Could you check a few things on this model? Use its own coordinates, in mm. A direction names the side the tool comes from. Give positions to 0.01 mm unless a question says otherwise; leave off trailing zeros. Order: outer loops, then holes, each group sorted by start corner. A loop starts at its lowest first (then second) coordinate and runs counter-clockwise, first axis right, second up. Notation, with made-up numbers: (48.25, 76.25) - (86.25, 76.25) arc R13 cw to (86.25, 101.25) - close; hole circle Ø9 at (56, 2). An arc over 180 degrees is marked (long way). Put each result on its own line as item: value.
from build123d import *

# Parameters (mm, degrees)
BOSS_EXTRUDE1_DEPTH     = 2.5
SKETCH2_R               = 10
BOSS_EXTRUDE2_DEPTH     = 15
CUT_EXTRUDE1_DEPTH      = 101.496505017
CUT_EXTRUDE1_DEPTH_BACK = 2.5
SKETCH3_R               = 7.5
BOSS_EXTRUDE3_START     = 2.5
SKETCH4_R               = 7.5
BOSS_EXTRUDE3_DEPTH     = 2.5


with BuildPart() as part:
    # Sketch1 → Boss-Extrude1 (new body)
    with BuildSketch(Plane(origin=(0, 0, 0), x_dir=(1, 0, 0), z_dir=(0, 1, 0))):
        with BuildLine():
            Line((-18.295454545, 4.75), (93.704545455, 4.75))
            ThreePointArc((93.704545455, 4.75), (98.454545455, 0), (93.704545455, -4.75))
            Line((93.704545455, -4.75), (-18.295454545, -4.75))
            ThreePointArc((-18.295454545, -4.75), (-23.045454545, 0), (-18.295454545, 4.75))
        make_face()
    extrude(amount=BOSS_EXTRUDE1_DEPTH)

    # Sketch2 → Boss-Extrude2 (add)
    with BuildSketch(Plane(origin=(0, 2.5, 0), x_dir=(1, 0, 0), z_dir=(0, 1, 0))):
        with Locations(Location((-12.795454545, 0, 0), (0, 0, 28.359350028))):
            Circle(SKETCH2_R)
    extrude(amount=BOSS_EXTRUDE2_DEPTH)

    # Sketch3 → Cut-Extrude1 (cut, two sides: drawn at the far end of the back side and taken through both)
    with BuildSketch(Plane(origin=(0, 17.5, 0), x_dir=(1, 0, 0), z_dir=(0, 1, 0)).offset(-CUT_EXTRUDE1_DEPTH_BACK)):
        with Locations(Location((-12.795454545, 0, 0), (0, 0, 90))):
            Circle(SKETCH3_R)
    extrude(amount=CUT_EXTRUDE1_DEPTH + CUT_EXTRUDE1_DEPTH_BACK, mode=Mode.SUBTRACT)

    # Sketch4 → Boss-Extrude3 (add)
    with BuildSketch(Plane(origin=(0, 15, 0), x_dir=(1, 0, 0), z_dir=(0, 1, 0)).offset(BOSS_EXTRUDE3_START)):
        with Locations((-12.795454545, 0)):
            Circle(SKETCH4_R)
    extrude(amount=-BOSS_EXTRUDE3_DEPTH)


solid = part.part
1) Suppose I cut it at D-D, the plane z = -7. List the corners of the cut face in (x, y) for me.
Filled in:
outline: (-19.94, 2.5) - (-5.65, 2.5) - (-5.65, 17.5) - (-19.94, 17.5) - close
2) Suppose I cut it at C-C, the plane y = 13.75. List the corners of the cut face in (x, z) for me, and give its area (3 significant figures).
Filled in:
outline: circle Ø20 at (-12.8, 0)
area: 314 mm^2
3) Which directions (+Z, -Z, +X, -X, +Y, -Y) give clear straight access to the entire face, cutting with the end or side of a thin tool? Please do faces 1 (the cylindrical face through (-23.044, 1.232, 0.104)), 2 (the flat face through (39, 0, 0)).
Filled in:
face 1: -X, -Y
face 2: +Z, -Z, +X, -X, -Y
4) Suppose I cut it at B-B, the plane x = 44.5. List the corners of the cut face in (y, z) for me.
Filled in:
outline: (0, -4.75) - (2.5, -4.75) - (2.5, 4.75) - (0, 4.75) - close
5) Suppose I cut it at A-A, the plane z = 0. List the corners of the cut face in (x, y) for me.
Filled in:
outline: (-23.05, 0) - (98.45, 0) - (98.45, 2.5) - (-2.8, 2.5) - (-2.8, 17.5) - (-22.8, 17.5) - (-22.8, 2.5) - (-23.05, 2.5) - close
6) I'm going to push flat-ended pins straight in: pin 1 (3 mm diameter, centred on x = 67.5, z = -1, fed in from +Y); pin 2 (2.5 mm diameter, centred on x = -17.5, z = 6.5, fed in from -Y); pin 3 (3 mm diameter, centred on x = 58.5, y = 1.5, fed in from +Z). Where does each tip first touch, or does it pass through?
Filled in:
pin 1: stops at y = 2.5
pin 2: stops at y = 2.5
pin 3: stops at z = 4.75
7) If I drill on line 1 (X direction, y = 12, z = -0.5); line 2 (Y direction, x = 48, z = -0.75); line 3 (Y direction, x = -15.5, z = -8), over which ranges is the centre line in solid material (lowest first)? Write a range as [from, to].
Filled in:
line 1: x = [-22.78, -2.81]
line 2: y = [0, 2.5]
line 3: y = [2.5, 17.5]
